Build history of the part. All positions in model axes, mm. A direction names the side the tool comes from. Give positions to 0.01 mm unless a question says otherwise; leave off trailing zeros. Order: outer loops, then holes, each group sorted by start corner. A loop starts at its lowest first (then second) coordinate and runs counter-clockwise, first axis right, second up. Notation, with made-up numbers: M -0.5,-6 L 55.5,-6 A32 cw 55.5,21 Z; hole C 34,60.5 d7. An arc over 180 degrees is marked long. One line per item, written item: value.
from build123d import *

# Parameters (mm, degrees)
RESSALTO_EXTRUS_O1_DEPTH        = 50
ESBO_O2_R                       = 1.6
CORTE_EXTRUS_O1_DEPTH           = 67.773947015
CORTE_EXTRUS_O2_DEPTH           = 8
CORTE_EXTRUS_O2_DRAFT           = -2
CORTE_EXTRUS_O2_PROFILE_2_DEPTH = 8
CORTE_EXTRUS_O2_PROFILE_2_DRAFT = -2
CORTE_EXTRUS_O2_PROFILE_3_DEPTH = 8
CORTE_EXTRUS_O2_PROFILE_3_DRAFT = -2
CORTE_EXTRUS_O2_PROFILE_4_DEPTH = 8
CORTE_EXTRUS_O2_PROFILE_4_DRAFT = -2
CORTE_EXTRUS_O2_PROFILE_5_DEPTH = 8
CORTE_EXTRUS_O2_PROFILE_5_DRAFT = -2
CORTE_EXTRUS_O2_PROFILE_6_DEPTH = 8
CORTE_EXTRUS_O2_PROFILE_6_DRAFT = -2
CORTE_EXTRUS_O2_PROFILE_7_DEPTH = 8
CORTE_EXTRUS_O2_PROFILE_7_DRAFT = -2
CORTE_EXTRUS_O2_PROFILE_8_DEPTH = 8
CORTE_EXTRUS_O2_PROFILE_8_DRAFT = -2


with BuildPart() as part:
    # Esboço1 → Ressalto-extrusão1 (new body)
    with BuildSketch(Plane.XY):
        with BuildLine():
            Line((0, 17.4), (0, -17.4))
            ThreePointArc((0, -17.4), (-7.6, -25), (0, -32.6))
            Line((0, -32.6), (0, -42.6))
            Line((0, -42.6), (-4, -42.6))
            Line((-4, -42.6), (-4, -36.313708499))
            ThreePointArc((-4, -36.313708499), (-9.797958971, -31.92820323), (-12, -25))
            Line((-12, -25), (-12, 25))
            ThreePointArc((-12, 25), (-9.797958971, 31.92820323), (-4, 36.313708499))
            Line((-4, 36.313708499), (-4, 42.6))
            Line((-4, 42.6), (0, 42.6))
            Line((0, 42.6), (0, 32.6))
            ThreePointArc((0, 32.6), (-7.6, 25), (0, 17.4))
        make_face()
    extrude(amount=RESSALTO_EXTRUS_O1_DEPTH)

    # Esboço2 → Corte-extrusão1 (cut, through all)
    with BuildSketch(Plane(origin=(0, 0, 0), x_dir=(0, 0, -1), z_dir=(1, 0, 0))):
        with Locations(Location((-42.5, 35, 0), (0, 0, 90))):
            Circle(ESBO_O2_R)
        with Locations(Location((-7.5, 35, 0), (0, 0, 90))):
            Circle(ESBO_O2_R)
        with Locations(Location((-7.5, -35, 0), (0, 0, 90))):
            Circle(ESBO_O2_R)
        with Locations(Location((-42.5, -35, 0), (0, 0, 90))):
            Circle(ESBO_O2_R)
        with Locations(Location((-42.5, -15, 0), (0, 0, 90))):
            Circle(ESBO_O2_R)
        with Locations(Location((-42.5, 15, 0), (0, 0, 90))):
            Circle(ESBO_O2_R)
        with Locations(Location((-7.5, 15, 0), (0, 0, 90))):
            Circle(ESBO_O2_R)
        with Locations(Location((-7.5, -15, 0), (0, 0, 90))):
            Circle(ESBO_O2_R)
    extrude(amount=-CORTE_EXTRUS_O1_DEPTH, mode=Mode.SUBTRACT)


with BuildPart() as corte_extrus_o2_tool:
    # Esboço3 → Corte-extrusão2 (with draft: the straight prism first)
    with BuildSketch(Plane.ZY.offset(12)):
        Polygon((10.25, 36.58771324), (7.5, 38.175426481), (4.75, 36.58771324), (4.75, 33.41228676), (7.5, 31.824573519), (10.25, 33.41228676), align=None)
    extrude(amount=-CORTE_EXTRUS_O2_DEPTH)
    # Corte-extrusão2: the draft: its side faces are tilted about the plane it starts from
    corte_extrus_o2_sides = [corte_extrus_o2_tool.faces().sort_by_distance(p)[0] for p in [
        (-8, 37.38156986, 8.875),
        (-8, 37.38156986, 6.125),
        (-8, 35, 4.75),
        (-8, 32.61843014, 6.125),
        (-8, 32.61843014, 8.875),
        (-8, 35, 10.25),
    ]]
    draft(corte_extrus_o2_sides, Plane.ZY.offset(12), CORTE_EXTRUS_O2_DRAFT)


with BuildPart() as part_1:
    add(part.part)

    # Corte-extrusão2: cut by corte_extrus_o2_tool
    add(corte_extrus_o2_tool.part, mode=Mode.SUBTRACT)


with BuildPart() as corte_extrus_o2_profile_2_tool:
    # Esboço3 → Corte-extrusão2 profile 2 (with draft: the straight prism first)
    with BuildSketch(Plane.ZY.offset(12)):
        Polygon((45.25, 36.58771324), (42.5, 38.175426481), (39.75, 36.58771324), (39.75, 33.41228676), (42.5, 31.824573519), (45.25, 33.41228676), align=None)
    extrude(amount=-CORTE_EXTRUS_O2_PROFILE_2_DEPTH)
    # Corte-extrusão2 profile 2: the draft: its side faces are tilted about the plane it starts from
    corte_extrus_o2_profile_2_sides = [corte_extrus_o2_profile_2_tool.faces().sort_by_distance(p)[0] for p in [
        (-8, 37.38156986, 43.875),
        (-8, 37.38156986, 41.125),
        (-8, 35, 39.75),
        (-8, 32.61843014, 41.125),
        (-8, 32.61843014, 43.875),
        (-8, 35, 45.25),
    ]]
    draft(corte_extrus_o2_profile_2_sides, Plane.ZY.offset(12), CORTE_EXTRUS_O2_PROFILE_2_DRAFT)


with BuildPart() as part_2:
    add(part_1.part)

    # Corte-extrusão2 profile 2: cut by corte_extrus_o2_profile_2_tool
    add(corte_extrus_o2_profile_2_tool.part, mode=Mode.SUBTRACT)


with BuildPart() as corte_extrus_o2_profile_3_tool:
    # Esboço3 → Corte-extrusão2 profile 3 (with draft: the straight prism first)
    with BuildSketch(Plane.ZY.offset(12)):
        Polygon((45.25, 16.58771324), (42.5, 18.175426481), (39.75, 16.58771324), (39.75, 13.41228676), (42.5, 11.824573519), (45.25, 13.41228676), align=None)
    extrude(amount=-CORTE_EXTRUS_O2_PROFILE_3_DEPTH)
    # Corte-extrusão2 profile 3: the draft: its side faces are tilted about the plane it starts from
    corte_extrus_o2_profile_3_sides = [corte_extrus_o2_profile_3_tool.faces().sort_by_distance(p)[0] for p in [
        (-8, 17.38156986, 43.875),
        (-8, 17.38156986, 41.125),
        (-8, 15, 39.75),
        (-8, 12.61843014, 41.125),
        (-8, 12.61843014, 43.875),
        (-8, 15, 45.25),
    ]]
    draft(corte_extrus_o2_profile_3_sides, Plane.ZY.offset(12), CORTE_EXTRUS_O2_PROFILE_3_DRAFT)


with BuildPart() as part_3:
    add(part_2.part)

    # Corte-extrusão2 profile 3: cut by corte_extrus_o2_profile_3_tool
    add(corte_extrus_o2_profile_3_tool.part, mode=Mode.SUBTRACT)


with BuildPart() as corte_extrus_o2_profile_4_tool:
    # Esboço3 → Corte-extrusão2 profile 4 (with draft: the straight prism first)
    with BuildSketch(Plane.ZY.offset(12)):
        Polygon((10.25, 16.58771324), (7.5, 18.175426481), (4.75, 16.58771324), (4.75, 13.41228676), (7.5, 11.824573519), (10.25, 13.41228676), align=None)
    extrude(amount=-CORTE_EXTRUS_O2_PROFILE_4_DEPTH)
    # Corte-extrusão2 profile 4: the draft: its side faces are tilted about the plane it starts from
    corte_extrus_o2_profile_4_sides = [corte_extrus_o2_profile_4_tool.faces().sort_by_distance(p)[0] for p in [
        (-8, 17.38156986, 8.875),
        (-8, 17.38156986, 6.125),
        (-8, 15, 4.75),
        (-8, 12.61843014, 6.125),
        (-8, 12.61843014, 8.875),
        (-8, 15, 10.25),
    ]]
    draft(corte_extrus_o2_profile_4_sides, Plane.ZY.offset(12), CORTE_EXTRUS_O2_PROFILE_4_DRAFT)


with BuildPart() as part_4:
    add(part_3.part)

    # Corte-extrusão2 profile 4: cut by corte_extrus_o2_profile_4_tool
    add(corte_extrus_o2_profile_4_tool.part, mode=Mode.SUBTRACT)


with BuildPart() as corte_extrus_o2_profile_5_tool:
    # Esboço3 → Corte-extrusão2 profile 5 (with draft: the straight prism first)
    with BuildSketch(Plane.ZY.offset(12)):
        Polygon((10.25, -13.41228676), (7.5, -11.824573519), (4.75, -13.41228676), (4.75, -16.58771324), (7.5, -18.175426481), (10.25, -16.58771324), align=None)
    extrude(amount=-CORTE_EXTRUS_O2_PROFILE_5_DEPTH)
    # Corte-extrusão2 profile 5: the draft: its side faces are tilted about the plane it starts from
    corte_extrus_o2_profile_5_sides = [corte_extrus_o2_profile_5_tool.faces().sort_by_distance(p)[0] for p in [
        (-8, -12.61843014, 8.875),
        (-8, -12.61843014, 6.125),
        (-8, -15, 4.75),
        (-8, -17.38156986, 6.125),
        (-8, -17.38156986, 8.875),
        (-8, -15, 10.25),
    ]]
    draft(corte_extrus_o2_profile_5_sides, Plane.ZY.offset(12), CORTE_EXTRUS_O2_PROFILE_5_DRAFT)


with BuildPart() as part_5:
    add(part_4.part)

    # Corte-extrusão2 profile 5: cut by corte_extrus_o2_profile_5_tool
    add(corte_extrus_o2_profile_5_tool.part, mode=Mode.SUBTRACT)


with BuildPart() as corte_extrus_o2_profile_6_tool:
    # Esboço3 → Corte-extrusão2 profile 6 (with draft: the straight prism first)
    with BuildSketch(Plane.ZY.offset(12)):
        Polygon((10.25, -33.41228676), (7.5, -31.824573519), (4.75, -33.41228676), (4.75, -36.58771324), (7.5, -38.175426481), (10.25, -36.58771324), align=None)
    extrude(amount=-CORTE_EXTRUS_O2_PROFILE_6_DEPTH)
    # Corte-extrusão2 profile 6: the draft: its side faces are tilted about the plane it starts from
    corte_extrus_o2_profile_6_sides = [corte_extrus_o2_profile_6_tool.faces().sort_by_distance(p)[0] for p in [
        (-8, -32.61843014, 8.875),
        (-8, -32.61843014, 6.125),
        (-8, -35, 4.75),
        (-8, -37.38156986, 6.125),
        (-8, -37.38156986, 8.875),
        (-8, -35, 10.25),
    ]]
    draft(corte_extrus_o2_profile_6_sides, Plane.ZY.offset(12), CORTE_EXTRUS_O2_PROFILE_6_DRAFT)


with BuildPart() as part_6:
    add(part_5.part)

    # Corte-extrusão2 profile 6: cut by corte_extrus_o2_profile_6_tool
    add(corte_extrus_o2_profile_6_tool.part, mode=Mode.SUBTRACT)


with BuildPart() as corte_extrus_o2_profile_7_tool:
    # Esboço3 → Corte-extrusão2 profile 7 (with draft: the straight prism first)
    with BuildSketch(Plane.ZY.offset(12)):
        Polygon((45.25, -33.41228676), (42.5, -31.824573519), (39.75, -33.41228676), (39.75, -36.58771324), (42.5, -38.175426481), (45.25, -36.58771324), align=None)
    extrude(amount=-CORTE_EXTRUS_O2_PROFILE_7_DEPTH)
    # Corte-extrusão2 profile 7: the draft: its side faces are tilted about the plane it starts from
    corte_extrus_o2_profile_7_sides = [corte_extrus_o2_profile_7_tool.faces().sort_by_distance(p)[0] for p in [
        (-8, -32.61843014, 43.875),
        (-8, -32.61843014, 41.125),
        (-8, -35, 39.75),
        (-8, -37.38156986, 41.125),
        (-8, -37.38156986, 43.875),
        (-8, -35, 45.25),
    ]]
    draft(corte_extrus_o2_profile_7_sides, Plane.ZY.offset(12), CORTE_EXTRUS_O2_PROFILE_7_DRAFT)


with BuildPart() as part_7:
    add(part_6.part)

    # Corte-extrusão2 profile 7: cut by corte_extrus_o2_profile_7_tool
    add(corte_extrus_o2_profile_7_tool.part, mode=Mode.SUBTRACT)


with BuildPart() as corte_extrus_o2_profile_8_tool:
    # Esboço3 → Corte-extrusão2 profile 8 (with draft: the straight prism first)
    with BuildSketch(Plane.ZY.offset(12)):
        Polygon((45.25, -13.41228676), (42.5, -11.824573519), (39.75, -13.41228676), (39.75, -16.58771324), (42.5, -18.175426481), (45.25, -16.58771324), align=None)
    extrude(amount=-CORTE_EXTRUS_O2_PROFILE_8_DEPTH)
    # Corte-extrusão2 profile 8: the draft: its side faces are tilted about the plane it starts from
    corte_extrus_o2_profile_8_sides = [corte_extrus_o2_profile_8_tool.faces().sort_by_distance(p)[0] for p in [
        (-8, -12.61843014, 43.875),
        (-8, -12.61843014, 41.125),
        (-8, -15, 39.75),
        (-8, -17.38156986, 41.125),
        (-8, -17.38156986, 43.875),
        (-8, -15, 45.25),
    ]]
    draft(corte_extrus_o2_profile_8_sides, Plane.ZY.offset(12), CORTE_EXTRUS_O2_PROFILE_8_DRAFT)


with BuildPart() as part_8:
    add(part_7.part)

    # Corte-extrusão2 profile 8: cut by corte_extrus_o2_profile_8_tool
    add(corte_extrus_o2_profile_8_tool.part, mode=Mode.SUBTRACT)


solid = part_8.part
1) Tool access for faces 1 (the face through (-4, -16, 9)), 2 (the face through (-6, 1, 50)): list every direction of +Z, -Z, +X, -X, +Y, -Y with a clear straight run to the whole face (end or side of a thin tool).
Check values:
face 1: -X
face 2: +Z, +X, -X, +Y, -Y
2) Saw through at C-C, the plane z = 36. Write the cut outline in (x, y), then the cut area to 3 significant figures.
Check values:
outline: M -12,-25 A12 ccw -4,-36.31 L -4,-42.6 L 0,-42.6 L 0,-32.6 A7.6 cw 0,-17.4 L 0,17.4 A7.6 cw 0,32.6 L 0,42.6 L -4,42.6 L -4,36.31 A12 ccw -12,25 Z
area: 691 mm^2
3) Saw through at D-D, the plane y = 35. Write the cut outline in (x, z), then the cut area to 3 significant figures.
Check values:
outline: M -6.63,0 L 0,0 L 0,5.9 L -4,5.9 L -4,5.03 L -6.63,4.94 Z; M -6.63,10.06 L -4,9.97 L -4,9.1 L 0,9.1 L 0,40.9 L -4,40.9 L -4,40.03 L -6.63,39.94 Z; M -6.63,45.06 L -4,44.97 L -4,44.1 L 0,44.1 L 0,50 L -6.63,50 Z
area: 280 mm^2
4) Drill centre lines: probe 1 along Z at (x, y) = (-1.4, -15); probe 2 along Y at (x, z) = (-2.5, 26); probe 3 along Y at (x, z) = (-1.5, 29.5). Where is each one in solid material? Low to high. Write a range as from..to.
Check values:
probe 1: 0..5.9, 9.1..40.9, 44.1..50
probe 2: -42.6..-32.18, -17.82..17.82, 32.18..42.6
probe 3: -42.6..-32.45, -17.55..17.55, 32.45..42.6
5) Saw through at A-A, the plane y = 15. Write the cut outline in (x, z), then the cut area to 3 significant figures.
Check values:
outline: M -12,0 L 0,0 L 0,5.9 L -4,5.9 L -4,5.03 L -12,4.75 Z; M -12,10.25 L -4,9.97 L -4,9.1 L 0,9.1 L 0,40.9 L -4,40.9 L -4,40.03 L -12,39.75 Z; M -12,45.25 L -4,44.97 L -4,44.1 L 0,44.1 L 0,50 L -12,50 Z
area: 491 mm^2
6) Pin check, flat tips, straight feed: pin 1 (4 mm diameter, centred on y = 35, z = 7.5, fed in from +X); pin 2 (1 mm diameter, centred on x = -7, z = 28.5, fed in from -Y); pin 3 (1.9 mm diameter, centred on y = 35, z = 42.5, fed in from -X); pin 4 (1 mm diameter, centred on x = -9, z = 20.5, fed in from +Y). Stop position of each tip, or through.
Check values:
pin 1: x = 0
pin 2: y = -35.09
pin 3: through
pin 4: y = 33.47
7) Saw through at B-B, the plane x = -1.25. Give the number of separate pieces and of enclosed holes in the cut face, then the cut area to 3 significant figures.
Check values:
separate pieces: 3
enclosed holes: 8
area: 2,700 mm^2
